```python
from build123d import *

# Parameters (mm, degrees)
SKETCH2_R           = 10
BOSS_EXTRUDE1_DEPTH = 15
SKETCH3_R           = 7.5
BOSS_EXTRUDE2_DEPTH = 10
SKETCH4_R           = 7.5
BOSS_EXTRUDE3_DEPTH = 30
SKETCH5_W           = 70
SKETCH5_H           = 80
CUT_EXTRUDE1_DEPTH  = 15
SKETCH6_W           = 35
SKETCH6_H           = 315


with BuildPart() as part:
    # Sketch1 → Revolve1 (revolve)
    with BuildSketch(Plane.XY):
        Polygon((0, 400), (50, 400), (50, 370), (45, 370), (45, 320), (40, 320), (40, 0), (22.5, 0), (22.5, 5), (35, 5), (35, 385), (0, 385), align=None)
    revolve(axis=Axis((0, -64.336492891, 0), (0, 1, 0)))

    # Sketch2 → Boss-Extrude1 (add, symmetric)
    with BuildSketch(Plane.XY):
        with BuildLine():
            Line((-30, 400), (30, 400))
            Line((30, 400), (19.138857956, 435.805524623))
            ThreePointArc((19.138857956, 435.805524623), (0, 450), (-19.138857956, 435.805524623))
            Line((-19.138857956, 435.805524623), (-30, 400))
        make_face()
        with Locations((0, 430)):
            Circle(SKETCH2_R, mode=Mode.SUBTRACT)
    extrude(amount=BOSS_EXTRUDE1_DEPTH, both=True)

    # Sketch3 → Boss-Extrude2 (add, symmetric)
    with BuildSketch(Plane.XY):
        with BuildLine():
            Line((30, 15), (30, 55))
            Line((30, 55), (62.373967528, 49.810951292))
            ThreePointArc((62.373967528, 49.810951292), (75, 35), (62.373967528, 20.189048708))
            Line((62.373967528, 20.189048708), (30, 15))
        make_face()
        with Locations((60, 35)):
            Circle(SKETCH3_R, mode=Mode.SUBTRACT)
    boss_extrude2 = extrude(amount=BOSS_EXTRUDE2_DEPTH, both=True)

    # Mirror1: Boss-Extrude2 across plane
    add(boss_extrude2.mirror(Plane(origin=(0, 0, 0), x_dir=(0, 0, 1), z_dir=(1, 0, 0))))

    # Sketch4 → Boss-Extrude3 (add, symmetric)
    with BuildSketch(Plane.XY):
        with BuildLine():
            Line((20, 250), (20, 190))
            Line((20, 190), (82.041582998, 195.08350067))
            ThreePointArc((82.041582998, 195.08350067), (105, 220), (82.041582998, 244.91649933))
            Line((82.041582998, 244.91649933), (20, 250))
        make_face()
        with Locations((80, 220)):
            Circle(SKETCH4_R, mode=Mode.SUBTRACT)
    extrude(amount=BOSS_EXTRUDE3_DEPTH, both=True)

    # Sketch5 → Cut-Extrude1 (cut, symmetric)
    with BuildSketch(Plane.XY):
        with Locations((95, 220)):
            Rectangle(SKETCH5_W, SKETCH5_H)
    extrude(amount=CUT_EXTRUDE1_DEPTH, both=True, mode=Mode.SUBTRACT)

    # Sketch6 → Cut-Revolve1 (revolve, cut)
    with BuildSketch(Plane.XY):
        with Locations((17.5, 162.5)):
            Rectangle(SKETCH6_W, SKETCH6_H)
    revolve(axis=Axis((0, 320, 0), (0, -1, 0)), mode=Mode.SUBTRACT)


solid = part.part
```
The model under review builds one solid part; all positions refer to its coordinate system, in mm. A direction names the side the tool comes from. Coordinates: 2 decimals unless noted, no trailing zeros. Write each loop counter-clockwise with the first axis right and the second up, starting at its lowest first coordinate (ties: lowest second). Pieces come first, ordered by that corner, then holes. Notation, with made-up numbers: (52, -16) -> (103, -16) arc R23 cw to (103, 3) -> close; hole circle Ø1 at (58, 20). An arc over 180 degrees is marked (long way). One line per item, written item: value. Start each with the question number.
Q1. The part is to be moulded in two halves that separate along Z. For faces 5 (the face through (56, 220, 30)), 6 (the face through (60, 220, 0)), 7 (the face through (72, 220, 15)), 8 (the face through (-0.4, 419.8, -15)), say which applies: +Z half, -Z half, draft (parallel to the pull), parting line (faces both ways), or undercut.
Q2. Add section A-A, the plane y = 220. Give the boundary of the cut face in (x, z), then the cut area to 3 significant figures.
Q3. Clearance check with flat-ended pins moving along their axes: P1, Ø12, axis at y = 300.5, z = -38.5, coming from the +X side; P2, Ø15, axis at x = -4, y = 435, coming from the -Z side; P3, Ø8, axis at x = 19.5, y = 306.5, coming from the +Z side. State where each tip first meets the part, or that it passes through.
Q4. Add section D-D, the plane y = 430. Give the boundary of the cut face in (x, z), then the cut area to 3 significant figures.
Q5. To check wall thickness, follow probe 1 along Z at (x, y) = (-1.5, 35); probe 2 along Z at (x, y) = (0, 355); probe 3 along X at (y, z) = (22, 1). State the ranges of each line that lie inside material, in increasing order.
Q6. Add section C-C, the plane y = 74. Give the boundary of the cut face in (x, z), then the cut area to 3 significant figures.
Q7. Add section B-B, the plane x = 0. Give the boundary of the cut face in (y, z).
Q8. For faces 1 (the face through (56, 220, -30)), 2 (the face through (-0.4, 419.8, 15)), 3 (the face through (-53, 31, 10)), 4 (the face through (47.69, 384.79, -15.02)), list the 3-axis set-ups (+Z, -Z, +X, -X, +Y, -Y) from which the entire face can be reached by the end or side of a thin tool; tool diameter is ignored.
Response:
1. face 5: +Z half
1. face 6: undercut
1. face 7: undercut
1. face 8: -Z half
2. outline: (26.46, -30) -> (72.5, -30) -> (72.5, -15) -> (60, -15) -> (60, 15) -> (72.5, 15) -> (72.5, 30) -> (26.46, 30) arc R40 ccw (long way) to start; (87.5, -30) -> (105, -30) -> (105, -15) -> (87.5, -15) -> close; (87.5, 15) -> (105, 15) -> (105, 30) -> (87.5, 30) -> close; hole circle Ø70 at (0, 0)
2. area: 3,530 mm²
3. P1: x = 23.32
3. P2: z = -15
3. P3: z = 36.87
4. outline: (-20.9, -15) -> (-10, -15) -> (-10, 15) -> (-20.9, 15) -> close; (10, -15) -> (20.9, -15) -> (20.9, 15) -> (10, 15) -> close
4. area: 654 mm²
5. probe 1: -39.97 to -34.97, 34.97 to 39.97
5. probe 2: -45 to -35, 35 to 45
5. probe 3: -67.48 to -34.99, 34.99 to 67.48
6. outline: circle Ø80 at (0, 0); hole circle Ø70 at (0, 0)
6. area: 1,180 mm²
7. outline: (0, -40) -> (320, -40) -> (320, -45) -> (370, -45) -> (370, -50) -> (400, -50) -> (400, -15) -> (420, -15) -> (420, 15) -> (400, 15) -> (400, 50) -> (370, 50) -> (370, 45) -> (320, 45) -> (320, 40) -> (0, 40) -> (0, 22.5) -> (5, 22.5) -> (5, 35) -> (385, 35) -> (385, -35) -> (5, -35) -> (5, -22.5) -> (0, -22.5) -> close; (440, -15) -> (450, -15) -> (450, 15) -> (440, 15) -> close
8. face 1: -Z, +X, -Y
8. face 2: +Z, +X, -X, +Y
8. face 3: +Z, -X, -Y
8. face 4: +Y
